Check sheet for the drawn part. Datum: minimum x, y, z corner. Units: mm. A direction names the side the tool comes from. Round coordinates to 2 decimals unless told otherwise and drop trailing zeros. Loops run counter-clockwise (first coordinate to the right, second up) from the corner with the lowest first, then second, coordinate; pieces in that order, holes last.
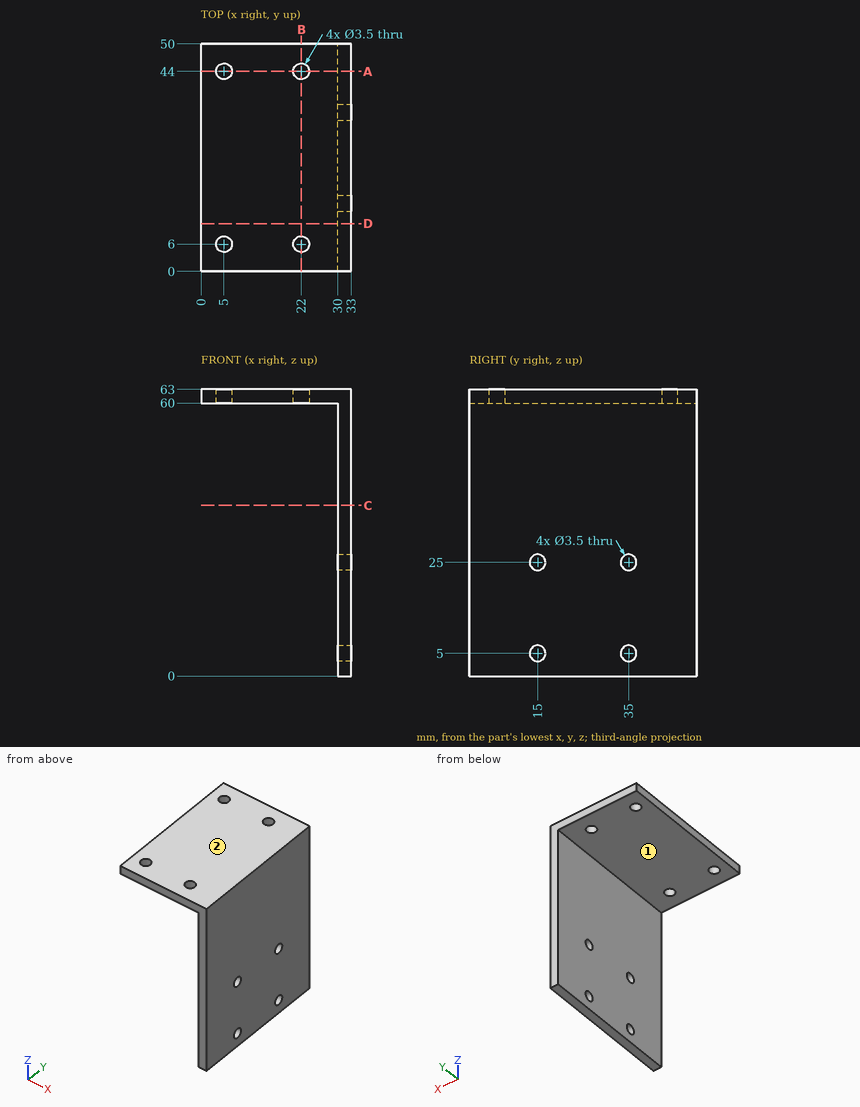
1) Sectioned sample at D-D, the plane y = 10.5. Record the cut outline in (x, z), then the cut area to 3 significant figures.
Report:
outline: (0, 60) - (30, 60) - (30, 0) - (33, 0) - (33, 63) - (0, 63) - close
area: 279 mm2
2) Gauge pin test, flat ends, axial feed: pin 1 (5.5 mm diameter, centred on y = 35, z = 5, fed in from -X); pin 2 (5.5 mm diameter, centred on x = 22, y = 44, fed in from -Z); pin 3 (4 mm diameter, centred on y = 35, z = 25, fed in from +X). Record the tip position at first contact, or that the pin passes through.
Report:
pin 1: stops at x = 30
pin 2: stops at z = 60
pin 3: stops at x = 33
3) Sectioned sample at C-C, the plane z = 37.5. Record the cut outline in (x, y), then the cut area to 3 significant figures.
Report:
outline: (30, 0) - (33, 0) - (33, 50) - (30, 50) - close
area: 150 mm2
4) Sectioned sample at A-A, the plane y = 44. Record the cut outline in (x, z), then the cut area to 3 significant figures.
Report:
outline: (0, 60) - (3.25, 60) - (3.25, 63) - (0, 63) - close; (6.75, 60) - (20.25, 60) - (20.25, 63) - (6.75, 63) - close; (23.75, 60) - (30, 60) - (30, 0) - (33, 0) - (33, 63) - (23.75, 63) - close
area: 258 mm2
5) Access from +Z, -Z, +X, -X, +Y, -Y to the whole of each face (thin tool, end or side, straight path). Record for the marked faces 1 and 2.
Report:
face 1: -Z, -X, +Y, -Y
face 2: +Z, +X, -X, +Y, -Y
6) Sectioned sample at B-B, the plane x = 22. Record the cut outline in (y, z).
Report:
outline: (0, 60) - (4.25, 60) - (4.25, 63) - (0, 63) - close; (7.75, 60) - (42.25, 60) - (42.25, 63) - (7.75, 63) - close; (45.75, 60) - (50, 60) - (50, 63) - (45.75, 63) - close
7) Scan lines: line 1 along Y through (x, z) = (31, 5); line 2 along Y through (x, z) = (22, 61.9); line 3 along Z through (x, y) = (26.5, 4). Record each from-to range of solid material in increasing order.
Report:
line 1: y = 0 to 13.25, 16.75 to 33.25, 36.75 to 50
line 2: y = 0 to 4.25, 7.75 to 42.25, 45.75 to 50
line 3: z = 60 to 63
